Could you check a few things on this drawing? It's one solid part, dimensions in mm from its lowest x, y, z. A direction names the side the tool comes from. Coordinates: 2 decimals unless noted, no trailing zeros. Write each loop counter-clockwise with the first axis right and the second up, starting at its lowest first coordinate (ties: lowest second). Pieces come first, ordered by that corner, then holes. Notation, with made-up numbers: (-22.75, -20) - (0.25, -20) arc R18 ccw to (0.25, 12) - close; hole circle Ø2 at (23, 72.5). An arc over 180 degrees is marked (long way). Answer as a JSON object with one key per item and string values. Group by question number.
1) On a 3-axis mill with a long thin cutter (end or side, diameter ignored), from which of +Z, -Z, +X, -X, +Y, -Y can I reach the whole of each face in a straight line? I mean the marked faces 1 and 2. Say none if no direction works.
2) If we section it at D-D (y = 56): Write out the boundary of the cut face in (x, z).
3) Will these pins go through, and if not, where does the flat tip stop? pin 1 Ø12 at (x, z) = (40, 28) entering from -Y; pin 2 Ø1.5 at (x, z) = (19.5, 15) entering from -Y.
4) Please list where these lines run through material, in increasing order: line 1 along X through (y, z) = (54, 25); line 2 along X through (y, z) = (60, 21.5); line 3 along Y through (x, z) = (59.5, 27.5).
5) If we section it at A-A (z = 25.4): Write out the boundary of the cut face in (x, y).
6) We'd pull the mould along Z, two halves only. Please class the marked faces 3, 4 and 5: released by +Z, released by -Z, zero draft, split by the parting line, or undercut.
7) If we section it at B-B (y = 25.4): Write out the boundary of the cut face in (x, z), plus the area to 3 significant figures.
8) If we section it at C-C (x = 74.5): Write out the boundary of the cut face in (y, z).
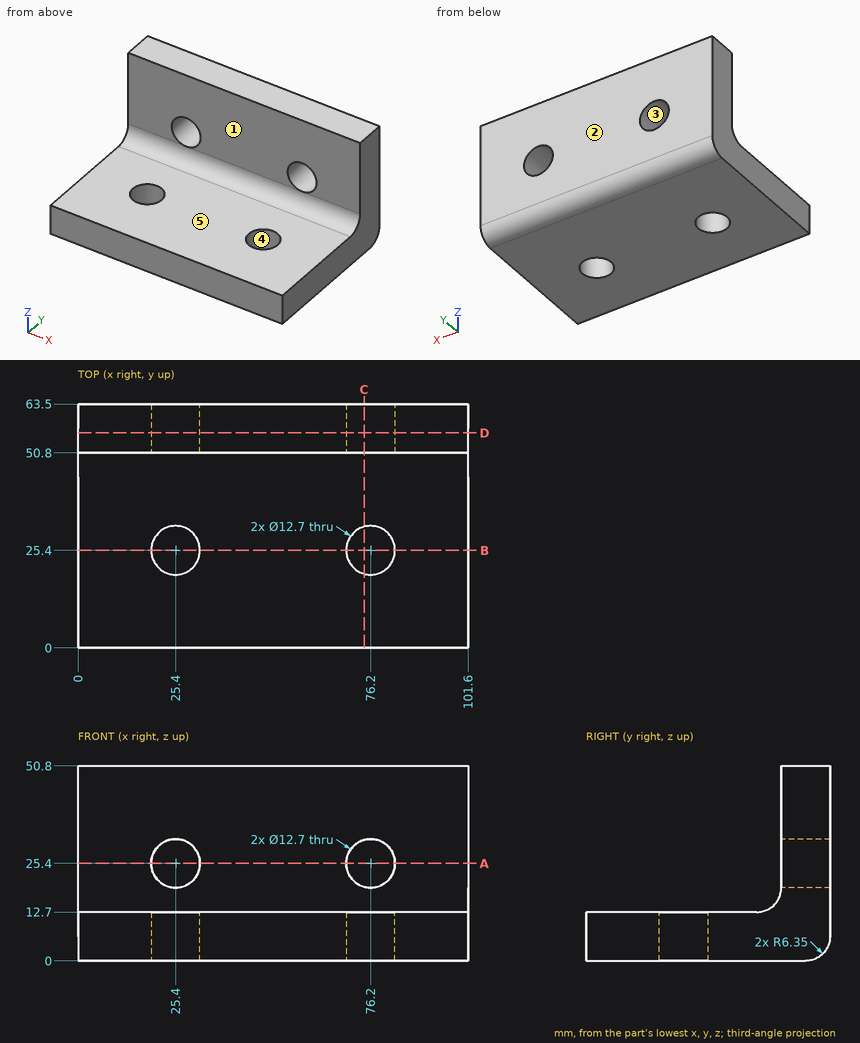
Here are the results:
{
 "1": {"face 1": "+Z, +X, -X, -Y", "face 2": "+Z, -Z, +X, -X, +Y"},
 "2": {"outline": "(0, 0) - (101.6, 0) - (101.6, 50.8) - (0, 50.8) - close; hole circle Ø12.7 at (25.4, 25.4); hole circle Ø12.7 at (76.2, 25.4)"},
 "3": {"pin 1": "stops at y = 50.8", "pin 2": "stops at y = 48.61"},
 "4": {"line 1": "x = 0 to 19.06, 31.74 to 69.86, 82.54 to 101.6", "line 2": "x = 0 to 20.39, 30.41 to 71.19, 81.21 to 101.6", "line 3": "y = 50.8 to 63.5"},
 "5": {"outline": "(0, 50.8) - (19.05, 50.8) - (19.05, 63.5) - (0, 63.5) - close; (31.75, 50.8) - (69.85, 50.8) - (69.85, 63.5) - (31.75, 63.5) - close; (82.55, 50.8) - (101.6, 50.8) - (101.6, 63.5) - (82.55, 63.5) - close"},
 "6": {"face 3": "undercut", "face 4": "zero draft", "face 5": "released by +Z"},
 "7": {"outline": "(0, 0) - (19.05, 0) - (19.05, 12.7) - (0, 12.7) - close; (31.75, 0) - (69.85, 0) - (69.85, 12.7) - (31.75, 12.7) - close; (82.55, 0) - (101.6, 0) - (101.6, 12.7) - (82.55, 12.7) - close", "area": "968 mm²"},
 "8": {"outline": "(0, 0) - (19.28, 0) - (19.28, 12.7) - (0, 12.7) - close; (31.52, 0) - (57.15, 0) arc R6.35 ccw to (63.5, 6.35) - (63.5, 19.28) - (50.8, 19.28) - (50.8, 19.05) arc R6.35 cw to (44.45, 12.7) - (31.52, 12.7) - close; (50.8, 31.52) - (63.5, 31.52) - (63.5, 50.8) - (50.8, 50.8) - close"}
}
